from build123d import *

# Parameters (mm, degrees)
SKETCH1_W           = 95
SKETCH1_H           = 75
BOSS_EXTRUDE1_DEPTH = 2
SKETCH2_W           = 95
SKETCH2_H           = 75
SKETCH2_W_2         = 91
SKETCH2_H_2         = 71
BOSS_EXTRUDE2_DEPTH = 35
SKETCH3_W           = 12.5
SKETCH3_H           = 12.5
CUT_EXTRUDE1_DEPTH  = 10
SKETCH4_W           = 12.5
SKETCH4_H           = 12.5
CUT_EXTRUDE2_DEPTH  = 10
SKETCH5_W           = 9.5
SKETCH5_H           = 5
CUT_EXTRUDE3_DEPTH  = 10
SKETCH6_W           = 15
SKETCH6_H           = 5
CUT_EXTRUDE4_DEPTH  = 10
SKETCH7_W           = 12
SKETCH7_H           = 7
CUT_EXTRUDE5_DEPTH  = 10
SKETCH8_W           = 91
SKETCH8_H           = 2
BOSS_EXTRUDE3_DEPTH = 3


with BuildPart() as part:
    # Sketch1 → Boss-Extrude1 (new body)
    with BuildSketch(Plane(origin=(0, 0, 0), x_dir=(1, 0, 0), z_dir=(0, 1, 0))):
        Rectangle(SKETCH1_W, SKETCH1_H)
    extrude(amount=BOSS_EXTRUDE1_DEPTH)

    # Sketch2 → Boss-Extrude2 (add)
    with BuildSketch(Plane(origin=(0, 2, 0), x_dir=(1, 0, 0), z_dir=(0, 1, 0))):
        Rectangle(SKETCH2_W, SKETCH2_H)
        with Locations((-0.148465207, 0)):
            Rectangle(SKETCH2_W_2, SKETCH2_H_2, mode=Mode.SUBTRACT)
    extrude(amount=BOSS_EXTRUDE2_DEPTH)

    # Sketch3 → Cut-Extrude1 (cut)
    with BuildSketch(Plane.XY.offset(37.5)):
        with Locations((-29.85, 15.25)):
            Rectangle(SKETCH3_W, SKETCH3_H)
    extrude(amount=-CUT_EXTRUDE1_DEPTH, mode=Mode.SUBTRACT)

    # Sketch4 → Cut-Extrude2 (cut)
    with BuildSketch(Plane.ZY.offset(47.5)):
        with Locations((-19.45, 15.25)):
            Rectangle(SKETCH4_W, SKETCH4_H)
    extrude(amount=-CUT_EXTRUDE2_DEPTH, mode=Mode.SUBTRACT)

    # Sketch5 → Cut-Extrude3 (cut)
    with BuildSketch(Plane.ZY.offset(47.5)):
        with Locations((14.55, 11.5)):
            Rectangle(SKETCH5_W, SKETCH5_H)
    extrude(amount=-CUT_EXTRUDE3_DEPTH, mode=Mode.SUBTRACT)

    # Sketch6 → Cut-Extrude4 (cut)
    with BuildSketch(Plane(origin=(0, 0, -37.5), x_dir=(-1, 0, 0), z_dir=(0, 0, -1))):
        with Locations((0, 2.5)):
            Rectangle(SKETCH6_W, SKETCH6_H)
    cut_extrude4 = extrude(amount=-CUT_EXTRUDE4_DEPTH, mode=Mode.SUBTRACT)

    # Mirror1: Cut-Extrude4 across plane
    add(cut_extrude4.mirror(Plane.XY), mode=Mode.SUBTRACT)

    # Sketch7 → Cut-Extrude5 (cut)
    with BuildSketch(Plane.ZY.offset(47.5)):
        with Locations((0, 3.5)):
            Rectangle(SKETCH7_W, SKETCH7_H)
    cut_extrude5 = extrude(amount=-CUT_EXTRUDE5_DEPTH, mode=Mode.SUBTRACT)

    # Mirror2: Cut-Extrude5 across plane
    add(cut_extrude5.mirror(Plane(origin=(0, 0, 0), x_dir=(0, 0, 1), z_dir=(1, 0, 0))), mode=Mode.SUBTRACT)

    # Sketch8 → Boss-Extrude3 (add)
    with BuildSketch(Plane.XY.offset(-35.5)):
        with Locations((-0.148465207, 12)):
            Rectangle(SKETCH8_W, SKETCH8_H)
    boss_extrude3 = extrude(amount=BOSS_EXTRUDE3_DEPTH)

    # Mirror3: Boss-Extrude3 across plane
    add(boss_extrude3.mirror(Plane.XY))


solid = part.part
Input: part model. Units: mm. Frame: model coordinates. A direction names the side the tool comes from. Coordinates: 2 decimals unless noted, no trailing zeros. Write each loop counter-clockwise with the first axis right and the second up, starting at its lowest first coordinate (ties: lowest second). Pieces come first, ordered by that corner, then holes. Notation, with made-up numbers: M -12,84.25 L 13,84.25 A24 cw 13,102.25 Z; hole C 70.5,36 d9. An arc over 180 degrees is marked long. Answer as a JSON object with one key per item and string values. Group by question number.
(1) Section B-B on x = -3.5. Output: boundary loops of the cut face in (y, z).
(2) Section A-A on z = 31. Output: boundary loops of the cut face in (x, y).
(3) Section D-D on x = -41. Output: boundary loops of the cut face in (y, z), plus the area to 3 significant figures.
(4) Mould query, pull axis Z, two halves, no side actions, for faces 6 (the face through (0, 5, -37)), 7 (the face through (-1, 18, -37.5)), 8 (the face through (-1, 11, 34)). Classes: pulls with the +Z half, pulls with the -Z half, needs draft (parallel to the pull), parting line crosses it, or undercut.
(5) Ray query, line 1 along X through (y, z) = (11.5, -7); line 2 along Z through (x, y) = (16.5, 26.5); line 3 along Z through (x, y) = (22, 12.5). Return the intervals inside material, ascending. Write a range as [from, to].
(6) Section C-C on z = 0. Output: boundary loops of the cut face in (x, y).
(7) Set-up query: faces 1 (the face through (-30, 21.5, 37)), 2 (the face through (44, 1, 6)), 3 (the face through (-44, 1, -6)), 4 (the face through (37.5, 1, 0)), 5 (the face through (-1, 12, -32.5)). Return all of +Z, -Z, +X, -X, +Y, -Y with unobstructed straight access to the full face (end or side cutting, diameter ignored); none if empty.
(8) Contact query for flat-ended pins moving along their axis: P1, Ø0.6, axis at y = 1.5, z = -0.5, coming from the +X side; P2, Ø1.6, axis at x = -3, y = 1, coming from the +Z side; P3, Ø1.6, axis at x = -1.5, z = -36.5, coming from the -Y side. Output: stop coordinate, or through.
Result set:
{
 "1": {"outline": "M 0,-27.5 L 2,-27.5 L 2,27.5 L 0,27.5 Z; M 5,-37.5 L 37,-37.5 L 37,-35.5 L 13,-35.5 L 13,-32.5 L 11,-32.5 L 11,-35.5 L 5,-35.5 Z; M 5,35.5 L 11,35.5 L 11,32.5 L 13,32.5 L 13,35.5 L 37,35.5 L 37,37.5 L 5,37.5 Z"},
 "2": {"outline": "M -47.5,0 L -7.5,0 L -7.5,2 L -45.65,2 L -45.65,37 L -47.5,37 Z; M 7.5,0 L 47.5,0 L 47.5,37 L 45.35,37 L 45.35,2 L 7.5,2 Z"},
 "3": {"outline": "M 0,-37.5 L 37,-37.5 L 37,-35.5 L 13,-35.5 L 13,-32.5 L 11,-32.5 L 11,-35.5 L 2,-35.5 L 2,-6 L 0,-6 Z; M 0,6 L 2,6 L 2,35.5 L 11,35.5 L 11,32.5 L 13,32.5 L 13,35.5 L 37,35.5 L 37,37.5 L 0,37.5 Z", "area": "278 mm2"},
 "4": {"face 6": "needs draft", "face 7": "pulls with the -Z half", "face 8": "undercut"},
 "5": {"line 1": "x = [-47.5, -45.65], [45.35, 47.5]", "line 2": "z = [-37.5, -35.5], [35.5, 37.5]", "line 3": "z = [-37.5, -32.5], [32.5, 37.5]"},
 "6": {"outline": "M -47.5,7 L -45.65,7 L -45.65,37 L -47.5,37 Z; M -37.5,0 L 37.5,0 L 37.5,2 L -37.5,2 Z; M 45.35,7 L 47.5,7 L 47.5,37 L 45.35,37 Z"},
 "7": {"face 1": "+Z", "face 2": "+X, -Y", "face 3": "-X, -Y", "face 4": "+X, +Y, -Y", "face 5": "+Y"},
 "8": {"P1": "stops at x = 37.5", "P2": "stops at z = 27.5", "P3": "stops at y = 5"}
}
